Could you check a few things on this model? Use its own coordinates, in mm. A direction names the side the tool comes from. Give positions to 0.01 mm unless a question says otherwise; leave off trailing zeros. Order: outer loops, then holes, each group sorted by start corner. A loop starts at its lowest first (then second) coordinate and runs counter-clockwise, first axis right, second up. Notation, with made-up numbers: (4, -30.5) -> (30, -30.5) arc R4 ccw to (30, -25.5) -> close; hole circle Ø6 at (87, -8.5). An arc over 180 degrees is marked (long way). Answer as CSV lines item,"result". Start each with the question number.
(1) I want a section at B-B (y = 0). Please give me the cut outline in (x, z).
(2) I want a section at A-A (z = -0.25). Please give me the cut outline in (x, y).
(3) On a 3-axis mill with a long thin cutter (end or side, diameter ignored), from which of +Z, -Z, +X, -X, +Y, -Y can I reach the whole of each face in a straight line? I mean faces 1 (the face through (3.94, -2.03, -2.85)), 2 (the face through (13, 0, 3)). Say none if no direction works.
(4) We'd pull the mould along Y, two halves only. Please class faces 3 (the face through (8, -1, 3)), 4 (the face through (14.51, 0.45, -2.15)), 5 (the face through (3.944, 3.484, -0.337)): released by +Y, released by -Y, zero draft, split by the parting line, or undercut.
(5) I need wall thicknesses on L1, parallel to Y at x = 12.5, z = 0; L2, parallel to X at y = 3, z = -1.25; L3, parallel to Y at x = 3, z = 0. Which ranges of each line are inside material? Lowest first, please.
(6) I want a section at C-C (x = 1.5). Please give me the cut outline in (y, z).
(7) Will these pins go through, and if not, where does the flat tip stop? pin 1 Ø1.5 at (x, z) = (9, 1) entering from +Y; pin 2 Ø4 at (x, y) = (14, 0.5) entering from +Z; pin 3 Ø1.5 at (x, z) = (10, 2) entering from +Y.
(8) I want a section at D-D (x = 10.25). Please give me the cut outline in (y, z).
```python
from build123d import *

# Parameters (mm, degrees)
EXTRUDE_1_DEPTH     = 8
SKETCH_2_R          = 3
EXTRUDE_2_DEPTH     = 10
SKETCH_3_R          = 2
CUT_EXTRUDE_1_DEPTH = 19.805177909
SKETCH_4_R          = 1.5
CUT_EXTRUDE_2_DEPTH = 10


with BuildPart() as part:
    # 草图1 → 凸台-拉伸1 (new body)
    with BuildSketch(Plane(origin=(0, 0, 0), x_dir=(0, 0, -1), z_dir=(1, 0, 0))):
        Polygon((1.704440109, -3.664453199), (4.025729616, -0.356138166), (2.321289507, 3.308315033), (-1.704440109, 3.664453199), (-4.025729616, 0.356138166), (-2.321289507, -3.308315033), align=None)
    extrude(amount=EXTRUDE_1_DEPTH)

    # 草图2 → 凸台-拉伸2 (add)
    with BuildSketch(Plane(origin=(8, 0, 0), x_dir=(0, 0, -1), z_dir=(1, 0, 0))):
        Circle(SKETCH_2_R)
    extrude(amount=EXTRUDE_2_DEPTH)

    # 草图3 → 切除-拉伸1 (cut, through all)
    with BuildSketch(Plane.ZY):
        Circle(SKETCH_3_R)
    extrude(amount=-CUT_EXTRUDE_1_DEPTH, mode=Mode.SUBTRACT)

    # 草图4 → 切除-拉伸2 (cut)
    with BuildSketch(Plane.XY):
        with Locations((13.078342884, 0)):
            Circle(SKETCH_4_R)
    extrude(amount=-CUT_EXTRUDE_2_DEPTH, mode=Mode.SUBTRACT)


solid = part.part
```
Final values:
1,outline,"(0, -3.86) -> (8, -3.86) -> (8, -3) -> (11.58, -3) -> (11.58, -2) -> (0, -2) -> close; (0, 2) -> (18, 2) -> (18, 3) -> (8, 3) -> (8, 3.86) -> (0, 3.86) -> close; (14.58, -3) -> (18, -3) -> (18, -2) -> (14.58, -2) -> close"
2,outline,"(0, -3.54) -> (8, -3.54) -> (8, -2.99) -> (18, -2.99) -> (18, -1.98) -> (0, -1.98) -> close; (0, 1.98) -> (18, 1.98) -> (18, 2.99) -> (8, 2.99) -> (8, 3.49) -> (0, 3.49) -> close"
3,face 1,"-Z, +X, -X, -Y"
3,face 2,"+X"
4,face 3,"zero draft"
4,face 4,"undercut"
4,face 5,"released by +Y"
5,L1,"-3 to -2, 2 to 3"
5,L2,"0 to 8"
5,L3,"-3.51 to -2, 2 to 3.51"
6,outline,"(-3.66, -1.7) -> (-0.36, -4.03) -> (3.31, -2.32) -> (3.66, 1.7) -> (0.36, 4.03) -> (-3.31, 2.32) -> close; hole circle Ø4 at (0, 0)"
7,pin 1,"y = 2.99"
7,pin 2,"z = 3"
7,pin 3,"y = 2.73"
8,outline,"circle Ø6 at (0, 0); hole circle Ø4 at (0, 0)"
